from build123d import *

# Parameters (mm, degrees)
F0_R     = 1.7272
F0_R_2   = 2.15265
F0_R_3   = 3.96875
F0_R_4   = 9.525
F0_R_5   = 7.9375
F1_DEPTH = 3.175
F2_R     = 4.7625


with BuildPart() as f1:
    # F0 (on Top) → F1 (new body)
    with BuildSketch(Plane.XY):
        with BuildLine():
            Line((-537.063671, 39.539974), (-588.318702, 20.884668))
            ThreePointArc((-588.318702, 20.884668), (-602.942304, 0), (-588.318702, -20.884668))
            Line((-588.318702, -20.884668), (-537.063671, -39.539974))
            Line((-537.063671, -39.539974), (-530.715026, -39.671139))
            Line((-530.715026, -39.671139), (-530.649444, -36.496817))
            Line((-530.649444, -36.496817), (-0.098374, -47.458199))
            Line((-0.098374, -47.458199), (-0.163957, -50.632521))
            Line((-0.163957, -50.632521), (24.301577, -51.721828))
            ThreePointArc((24.301577, -51.721828), (24.407469, -51.725363), (24.513413, -51.726541))
            Line((24.513413, -51.726541), (84.952916, -51.726541))
            Line((84.952916, -51.726541), (84.952916, 51.726541))
            Line((84.952916, 51.726541), (24.513413, 51.726541))
            ThreePointArc((24.513413, 51.726541), (24.407469, 51.725363), (24.301577, 51.721828))
            Line((24.301577, 51.721828), (-0.163957, 50.632521))
            Line((-0.163957, 50.632521), (-0.098374, 47.458199))
            Line((-0.098374, 47.458199), (-530.649444, 36.496817))
            Line((-530.649444, 36.496817), (-530.715026, 39.671139))
            Line((-530.715026, 39.671139), (-537.063671, 39.539974))
        make_face()
        with Locations((-516.266618, -32.030455)):
            Circle(F0_R, mode=Mode.SUBTRACT)
        with Locations((-592.503891, -11.786586)):
            Circle(F0_R_2, mode=Mode.SUBTRACT)
        with Locations((-568.930718, -11.786586)):
            Circle(F0_R_3, mode=Mode.SUBTRACT)
        with Locations((-14.284452, -42.401593)):
            Circle(F0_R, mode=Mode.SUBTRACT)
        with Locations((24.513413, -46.964041)):
            Circle(F0_R_2, mode=Mode.SUBTRACT)
        with Locations((80.190416, -46.964041)):
            Circle(F0_R_2, mode=Mode.SUBTRACT)
        with Locations((-11.786586, -11.786586)):
            Circle(F0_R_2, mode=Mode.SUBTRACT)
        with Locations((11.786586, -11.786586)):
            Circle(F0_R_2, mode=Mode.SUBTRACT)
        with Locations((-580.717304, 0)):
            Circle(F0_R_4, mode=Mode.SUBTRACT)
        with Locations((-529.917304, 0)):
            Circle(F0_R, mode=Mode.SUBTRACT)
        with Locations((-592.503891, 11.786586)):
            Circle(F0_R_3, mode=Mode.SUBTRACT)
        with Locations((-568.930718, 11.786586)):
            Circle(F0_R_2, mode=Mode.SUBTRACT)
        with Locations((-516.266618, 32.030455)):
            Circle(F0_R, mode=Mode.SUBTRACT)
        with Locations((-50.8, 0)):
            Circle(F0_R, mode=Mode.SUBTRACT)
        with Locations((-11.786586, 11.786586)):
            Circle(F0_R_2, mode=Mode.SUBTRACT)
        Circle(F0_R_5, mode=Mode.SUBTRACT)
        with Locations((11.786586, 11.786586)):
            Circle(F0_R_2, mode=Mode.SUBTRACT)
        with Locations((-14.284452, 42.401593)):
            Circle(F0_R, mode=Mode.SUBTRACT)
        with Locations((24.513413, 46.964041)):
            Circle(F0_R_2, mode=Mode.SUBTRACT)
        with Locations((80.190416, 46.964041)):
            Circle(F0_R_2, mode=Mode.SUBTRACT)
    extrude(amount=F1_DEPTH)

    # F2
    f2_edges = [f1.edges().sort_by_distance(p)[0] for p in [
        (84.952916, 51.726541, 1.5875),
        (84.952916, -51.726541, 1.5875),
    ]]
    fillet(f2_edges, radius=F2_R)


solid = f1.part
Could you check a few things on this model? Use its own coordinates, in mm. Round coordinates to 2 decimals unless told otherwise and drop trailing zeros. Order: outer loops, then holes, each group sorted by start corner. A loop starts at its lowest first (then second) coordinate and runs counter-clockwise, first axis right, second up. Notation, with made-up numbers: M 28.5,11 L 49.5,11 A17 ccw 49.5,23 Z; hole C 34,-16.5 d7. An arc over 180 degrees is marked long. One line per item, written item: value.
(1) Imagine slicing it at A-A (x = -300). Write out the boundary of the cut face in (y, z) (3 decimals).
Ans:
outline: M -41.262,0 L 41.262,0 L 41.262,3.175 L -41.262,3.175 Z
(2) I'm going to push flat-ended pins straight in: P1, Ø1, axis at x = -289.5, z = 2, coming from the -Y side; P2, Ø1, axis at x = -300.5, z = 0.5, coming from the +Y side. Where does each tip first touch, or does it pass through?
Ans:
P1: stops at y = -41.49
P2: stops at y = 41.26
(3) Imagine slicing it at B-B (z = 0.95). Count the separate pieces of the cut face and the enclosed holes in it, and give its area (3 significant figures).
Ans:
separate pieces: 1
enclosed holes: 20
area: 56,600 mm^2
(4) Imagine slicing it at C-C (x = -124.5). Write out the boundary of the cut face in (y, z) (3 decimals).
Ans:
outline: M -44.888,0 L 44.888,0 L 44.888,3.175 L -44.888,3.175 Z
(5) If we mould it in two halves opening along Y, with no side actions, what happens to faces 1 (the cylindrical face through (-1.72, -7.75, 1.57)), 2 (the cylindrical face through (-602.94, 0.38, 1.57)), 3 (the flat face through (-563, -30.1, 1.6)), 4 (the cylindrical face through (-571.63, 2.86, 1.57))? For each: released by +Y, released by -Y, zero draft, split by the parting line, or undercut.
Ans:
face 1: undercut
face 2: split by the parting line
face 3: released by -Y
face 4: undercut
(6) I need wall thicknesses on line 1 along Y through (x, z) = (0, 0.85); line 2 along X through (y, z) = (12, 1.3); line 3 along X through (y, z) = (13.5, 2.2). Which ranges of each line are inside material? Lowest first, please. Write a range as from..to.
Ans:
line 1: y = -50.64..-7.94, 7.94..50.64
line 2: x = -599.42..-596.47, -588.54..-571.07, -566.79..-13.93, -9.64..9.64, 13.93..84.95
line 3: x = -598.37..-596.08, -588.92..-570.23, -567.63..-13.09, -10.48..10.48, 13.09..84.95
